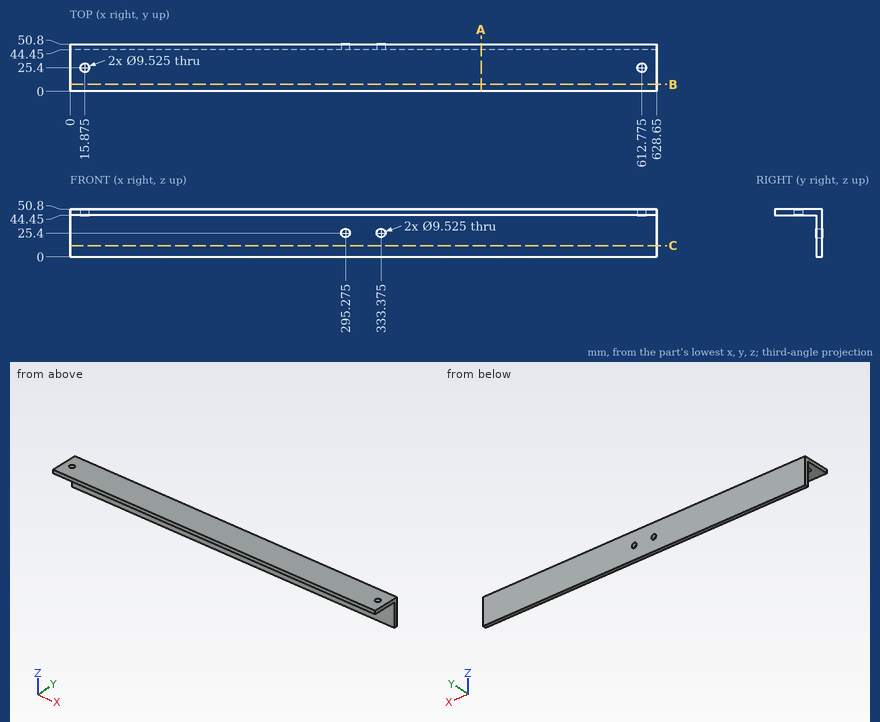
Print and shaded views of the part. All mm, measured from the part's lowest x, y and z. Give positions to 0.01 mm unless a question says otherwise; leave off trailing zeros. Loops run counter-clockwise (first coordinate to the right, second up) from the corner with the lowest first, then second, coordinate; pieces in that order, holes last. Notation, with made-up numbers: (33, 49) -> (46, 49) arc R16 cw to (46, 58) -> close; hole circle Ø2 at (29, 22.5). An arc over 180 degrees is marked (long way). Use a Markdown table: item, result.
1. Slice it at B-B (y = 7.5). List the corners of the cut face in (x, z).
Check result:
| item | result |
|---|---|
| outline | (0, 44.45) -> (628.65, 44.45) -> (628.65, 50.8) -> (0, 50.8) -> close |
2. Slice it at A-A (x = 440.5). List the corners of the cut face in (y, z).
Check result:
| item | result |
|---|---|
| outline | (0, 44.45) -> (44.45, 44.45) -> (44.45, 0) -> (50.8, 0) -> (50.8, 50.8) -> (0, 50.8) -> close |
3. Flat gauge pins, fed straight in: pin 1 (5 mm diameter, centred on y = 26, z = 42.5, fed in from -X); pin 2 (1.5 mm diameter, centred on x = 306, y = 35.5, fed in from -Z); pin 3 (12 mm diameter, centred on x = 399, z = 20.5, fed in from -Y). Where does each tip first touch, or does it go through?
Check result:
| item | result |
|---|---|
| pin 1 | stops at x = 0 |
| pin 2 | stops at z = 44.45 |
| pin 3 | stops at y = 44.45 |
4. Wall check: L1, parallel to X at y = 25, z = 47; L2, parallel to X at y = 48, z = 25; L3, parallel to Z at x = 485, y = 26. Give the ranges that are in metal, low to high. Write a range as [from, to].
Check result:
| item | result |
|---|---|
| L1 | x = [0, 11.13], [20.62, 608.03], [617.52, 628.65] |
| L2 | x = [0, 290.53], [300.02, 328.63], [338.12, 628.65] |
| L3 | z = [44.45, 50.8] |
